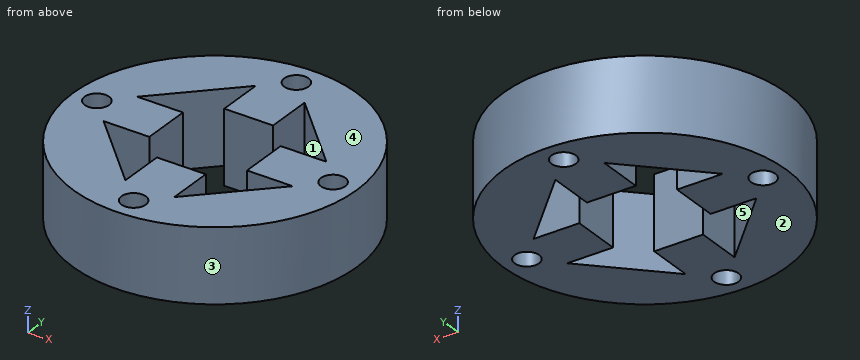
```python
from build123d import *

# Parameters (mm, degrees)
SKETCH6_R                 = 29
SKETCH6_R_2               = 20
INNER_RING_DEPTH          = 15
MOTOR_CONNECTOR_CUT_DEPTH = 15
SKETCH8_R                 = 2.5
M3_HOLES_DEPTH            = 38
M3_HOLES_DEPTH_BACK       = 53
BOSS_EXTRUDE1_DEPTH       = 15


with BuildPart() as part:
    # Sketch6 → Inner Ring (new body)
    with BuildSketch(Plane.XY):
        Circle(SKETCH6_R)
        Circle(SKETCH6_R_2, mode=Mode.SUBTRACT)
    extrude(amount=-INNER_RING_DEPTH)

    # Sketch7 → Motor Connector Cut (add)
    with BuildSketch(Plane.XY):
        with BuildLine():
            ThreePointArc((20, 0), (19.840593925, 2.52008585), (19.364916731, 5))
            Line((19.364916731, 5), (9.999996731, 5))
            Line((9.999996731, 5), (9.999996731, -5))
            Line((9.999996731, -5), (19.364916731, -5))
            ThreePointArc((19.364916731, -5), (19.840593925, -2.52008585), (20, 0))
        make_face()
        with BuildLine():
            ThreePointArc((5, 19.364916731), (0, 20), (-5, 19.364916731))
            Line((-5, 19.364916731), (-5, 9.999996731))
            Line((-5, 9.999996731), (5, 9.999996731))
            Line((5, 9.999996731), (5, 19.364916731))
        make_face()
        with BuildLine():
            Line((-9.999996731, -5), (-9.999996731, 5))
            Line((-9.999996731, 5), (-19.364916731, 5))
            ThreePointArc((-19.364916731, 5), (-20, 0), (-19.364916731, -5))
            Line((-19.364916731, -5), (-9.999996731, -5))
        make_face()
        with BuildLine():
            Line((-5, -9.999996731), (-5, -19.364916731))
            ThreePointArc((-5, -19.364916731), (0, -20), (5, -19.364916731))
            Line((5, -19.364916731), (5, -9.999996731))
            Line((5, -9.999996731), (-5, -9.999996731))
        make_face()
    extrude(amount=-MOTOR_CONNECTOR_CUT_DEPTH)

    # Sketch8 → M3 Holes (cut, two sides)
    with BuildSketch(Plane.XY) as m3_holes_sk:
        with Locations((0, 24.182458366)):
            Circle(SKETCH8_R)
        with Locations((24.182458366, 0)):
            Circle(SKETCH8_R)
        with Locations((0, -24.182458366)):
            Circle(SKETCH8_R)
        with Locations((-24.182458366, 0)):
            Circle(SKETCH8_R)
    extrude(amount=M3_HOLES_DEPTH, mode=Mode.SUBTRACT)
    extrude(m3_holes_sk.sketch, amount=-M3_HOLES_DEPTH_BACK, mode=Mode.SUBTRACT)

    # Sketch9 → Boss-Extrude1 (add)
    with BuildSketch(Plane(origin=(0, 0, -15), x_dir=(-1, 0, 0), z_dir=(0, 0, -1))):
        with BuildLine():
            Line((-19.364916731, 5), (-5, 19.364916731))
            ThreePointArc((-5, 19.364916731), (-14.142135624, 14.142135624), (-19.364916731, 5))
        make_face()
        with BuildLine():
            Line((5, 19.364916731), (19.364916731, 5))
            ThreePointArc((19.364916731, 5), (14.142135624, 14.142135624), (5, 19.364916731))
        make_face()
        with BuildLine():
            Line((19.364916731, -5), (5, -19.364916731))
            ThreePointArc((5, -19.364916731), (14.142135624, -14.142135624), (19.364916731, -5))
        make_face()
        with BuildLine():
            Line((-5, -19.364916731), (-19.364916731, -5))
            ThreePointArc((-19.364916731, -5), (-14.142135624, -14.142135624), (-5, -19.364916731))
        make_face()
    extrude(amount=-BOSS_EXTRUDE1_DEPTH)


solid = part.part
```
Can you work these out from the model? Positions are in its coordinate system, mm. Face numbers are marked on the shaded views. A direction names the side the tool comes from. Give positions to 0.01 mm unless a question says otherwise; leave off trailing zeros. Loops run counter-clockwise (first coordinate to the right, second up) from the corner with the lowest first, then second, coordinate; pieces in that order, holes last. Notation, with made-up numbers: M 59,25.25 L 65,25.25 A23 ccw 65,59.25 Z; hole C 61,35.5 d5. An arc over 180 degrees is marked long. Use one line per item in the form item = value. Start each with the question number.
(1) I want a section at C-C, the plane x = -25. Write out the boundary of the cut face in (y, z), and give its area (3 significant figures).
(2) On a 3-axis mill with a long thin cutter (end or side, diameter ignored), from which of +Z, -Z, +X, -X, +Y, -Y can I reach the whole of each face in a straight line? I mean the marked faces 1 and 2. Say none if no direction works.
(3) Please list where these lines run through material, in increasing order: line 1 (Y direction, x = 0, z = -11); line 2 (Y direction, x = 11, z = -1); line 3 (X direction, y = -15, z = -8).
(4) I'm going to push flat-ended pins straight in: P1, Ø3, axis at y = 13, z = -9.5, coming from the -X side; P2, Ø7.5, axis at y = -13.5, z = -8, coming from the +X side; P3, Ø3, axis at x = -14, z = -6.5, coming from the +Y side. Where does each tip first touch, or does it pass through?
(5) Thinking about a two-plate mould opening in X: for the marked faces 3, 4 and 5, which applies, released by +X, released by -X, zero draft, split by the parting line, or undercut?
(6) I want a section at D-D, the plane y = 16. Write out the boundary of the cut face in (x, z), and give its area (3 significant figures).
(7) I want a section at A-A, the plane x = 0. Write out the boundary of the cut face in (y, z), and give its area (3 significant figures).
Worked out:
q1.outline = M -14.7,-15 L -2.36,-15 L -2.36,0 L -14.7,0 Z; M 2.36,-15 L 14.7,-15 L 14.7,0 L 2.36,0 Z
q1.area = 370 mm²
q2.face_1 = +Z, -Z
q2.face_2 = -Z, +X, -X, +Y, -Y
q3.line_1 = -29 to -26.68, -21.68 to -10, 10 to 21.68, 26.68 to 29
q3.line_2 = -26.83 to -13.36, -5 to 5, 13.36 to 26.83
q3.line_3 = -24.82 to -9.36, -5 to 5, 9.36 to 24.82
q4.P1 = -26.62
q4.P2 = 27.31
q4.P3 = 26.17
q5.face_3 = split by the parting line
q5.face_4 = zero draft
q5.face_5 = undercut
q6.outline = M -24.19,-15 L -8.36,-15 L -8.36,0 L -24.19,0 Z; M -5,-15 L 5,-15 L 5,0 L -5,0 Z; M 8.36,-15 L 24.19,-15 L 24.19,0 L 8.36,0 Z
q6.area = 625 mm²
q7.outline = M -29,-15 L -26.68,-15 L -26.68,0 L -29,0 Z; M -21.68,-15 L -10,-15 L -10,0 L -21.68,0 Z; M 10,-15 L 21.68,-15 L 21.68,0 L 10,0 Z; M 26.68,-15 L 29,-15 L 29,0 L 26.68,0 Z
q7.area = 420 mm²
